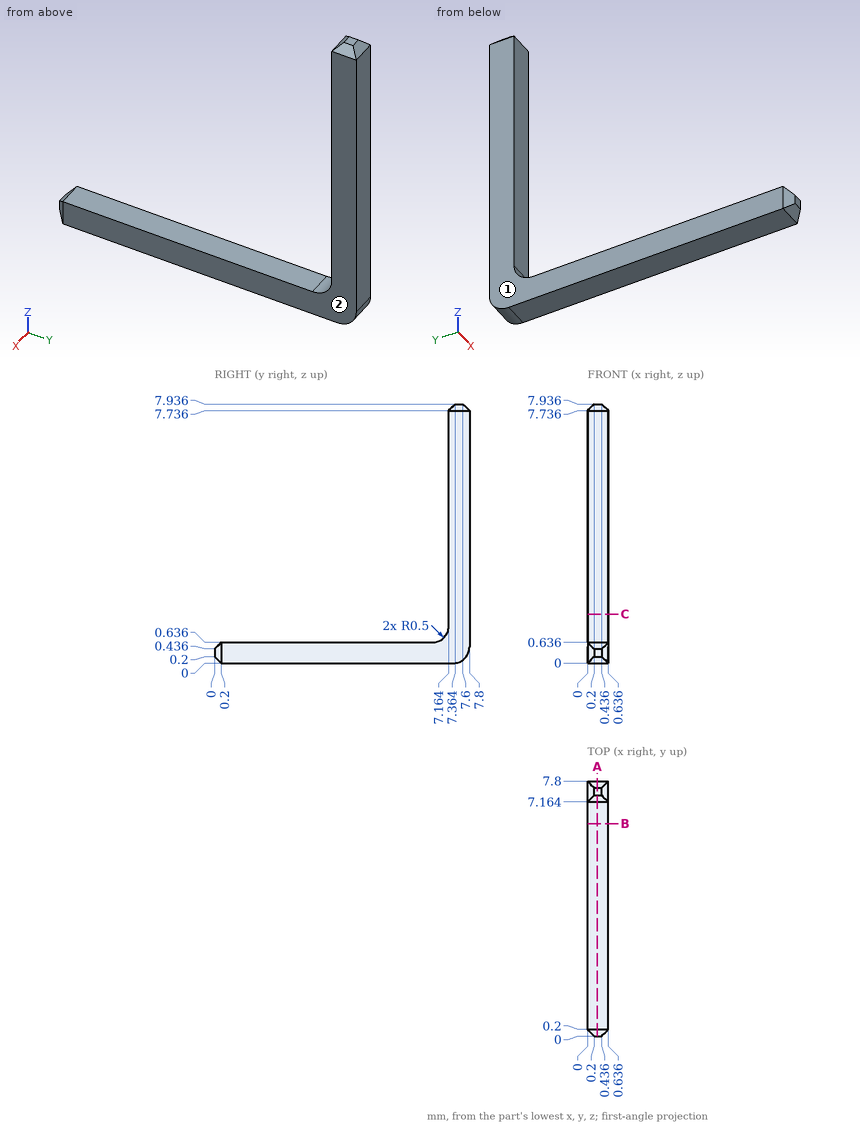
Geometry: see drawing. Coordinates: mm, zero at the bounding-box minimum. Give positions to 0.01 mm unless a question says otherwise; leave off trailing zeros. Loops run counter-clockwise (first coordinate to the right, second up) from the corner with the lowest first, then second, coordinate; pieces in that order, holes last. Notation, with made-up numbers: (3, 47.5) -> (58, 47.5) arc R30 ccw to (58, 77.5) -> close; hole circle Ø8 at (80, 7.25). An arc over 180 degrees is marked (long way). Use CSV: the item, a comma, the result in double quotes.
(1) Cut plane B-B (y = 6.5). Output: boundary loops of the cut face in (x, z).
From the geometry:
outline,"(0, 0) -> (0.64, 0) -> (0.64, 0.64) -> (0, 0.64) -> close"
(2) Pull-direction query (X, two-part tool) for the marked faces 1 and 2; classes: released by +X, released by -X, zero draft, split by the parting line, or undercut.
From the geometry:
face 1,"released by -X"
face 2,"released by +X"
(3) Cut plane A-A (x = 0.3). Output: boundary loops of the cut face in (y, z), plus the area to 3 significant figures.
From the geometry:
outline,"(0, 0.2) -> (0.2, 0) -> (7.3, 0) arc R0.5 ccw to (7.8, 0.5) -> (7.8, 7.74) -> (7.6, 7.94) -> (7.36, 7.94) -> (7.16, 7.74) -> (7.16, 1.14) arc R0.5 cw to (6.66, 0.64) -> (0.2, 0.64) -> (0, 0.44) -> close"
area,"9.52 mm^2"
(4) Ray query, line 1 along Z through (x, y) = (0.5, 5); line 2 along Y through (x, z) = (0.55, 5); line 3 along Y through (x, z) = (0.15, 1). Return the intervals inside material, ascending. Write a range as [from, to].
From the geometry:
line 1,"[0, 0.64]"
line 2,"[7.16, 7.8]"
line 3,"[7.15, 7.8]"
(5) First-contact query: P1, Ø1, axis at y = 3, z = 2.5, coming from the -X side. Flat tip, straight axial feed; report the tip coordinate or a pass-through.
From the geometry:
P1,"through"
(6) Cut plane C-C (z = 1.5). Output: boundary loops of the cut face in (x, y), plus the area to 3 significant figures.
From the geometry:
outline,"(0, 7.16) -> (0.64, 7.16) -> (0.64, 7.8) -> (0, 7.8) -> close"
area,"0.404 mm^2"
